Geometry: final body of the model. Coordinates: model frame, mm. Face numbers are marked on the shaded views. Give positions to 0.01 mm unless a question says otherwise; leave off trailing zeros. Order: outer loops, then holes, each group sorted by start corner. A loop starts at its lowest first (then second) coordinate and runs counter-clockwise, first axis right, second up. Notation, with made-up numbers: (-37.5, -14.5) - (-10.5, -14.5) arc R15 cw to (-10.5, -7.5) - close; hole circle Ø8 at (64.5, 41.5). An arc over 180 degrees is marked (long way). One line per item, written item: value.
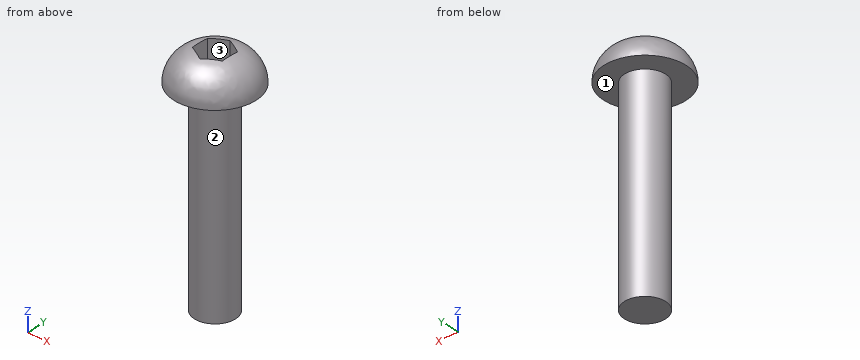
Autodesk Inventor part; units mm, degrees
ref_plane "YZ Plane" through (0, 0, 0) normal (1, 0, 0) x (0, 1, 0)
ref_plane "XZ Plane" through (0, 0, 0) normal (0, 1, 0) x (-1, 0, 0)
ref_plane "XY Plane" through (0, 0, 0) normal (0, 0, 1) x (1, 0, 0)
sketch "スケッチ1" plane through (0, 0, 0) normal (0, 0, 1) x (1, 0, 0)
  circle A0 centre (0, 0) radius 2
  dimension "d0" = 4
extrude "押し出し1" add sketch "スケッチ1" along normal blind 20
sketch "スケッチ2" plane through (0, 0, 20) normal (0, 0, 1) x (1, 0, 0)
  circle A0 centre (0, 0) radius 2
  circle A1 centre (0, 0) radius 4
  dimension "d3" = 8
extrude "押し出し2" add sketch "スケッチ2" along normal blind 3 contours A0 | A1
fillet "フィレット1" radius 3 1 edges at (-4, 0, 23)
thread "ねじ1"
sketch "スケッチ3" plane through (0, 0, 23) normal (0, 0, 1) x (1, 0, 0)
  line L0 (-1.5, 0.866) -> (0, 1.7321)
  line L1 (0, 1.7321) -> (1.5, 0.866)
  line L2 (1.5, 0.866) -> (1.5, -0.866)
  line L3 (1.5, -0.866) -> (0, -1.7321)
  line L4 (0, -1.7321) -> (-1.5, -0.866)
  line L5 (-1.5, -0.866) -> (-1.5, 0.866)
  point P0 (0, 0)
  point P1 (0, 0)
  point P2 (-1.5, 0)
  dimension "d9" = 3
extrude "押し出し3" cut sketch "スケッチ3" against normal blind 2
properties part number "SB　M4 8mm なべネジ" material "Stainless Steel, 440C"
1) Mould query, pull axis Y, two halves, no side actions, for the marked faces 1, 2 and 3. Classes: released by +Y, released by -Y, zero draft, split by the parting line, or undercut.
Answers below:
face 1: zero draft
face 2: split by the parting line
face 3: undercut
2) Section A-A, the plane z = 2. Return loops of the section in (x, y), then the cut area to 3 significant figures.
Answers below:
outline: circle Ø4 at (0, 0)
area: 12.6 mm^2
3) Material intervals for line 1 along Z through (x, y) = (0, -0.75); line 2 along Y through (x, z) = (-3.5, 20.75); line 3 along X through (y, z) = (0, 21.5), sorted ascending.
Answers below:
line 1: 0 to 21
line 2: -1.73 to 1.73
line 3: -3.6 to -1.5, 1.5 to 3.6
4) First-contact query: pin 1 (3 mm diameter, centred on x = -2.5, y = 3, fed in from +Z); pin 2 (0.5 mm diameter, centred on y = 0.5, z = 22, fed in from +X); pin 3 (3 mm diameter, centred on x = 3, z = 10, fed in from +Y). Flat tips, straight axial feed; report the tip coordinate or a pass-through.
Answers below:
pin 1: z = 22.65
pin 2: x = 3.4
pin 3: y = 1.32
